```python
from build123d import *

# Parameters (mm, degrees)
F0_R     = 9
F0_R_2   = 1.45
F1_DEPTH = 2
F2_R     = 3
F2_R_2   = 1.5
F3_DEPTH = 15
F5_SIZE2 = 5
F5_SIZE  = 1
F6_DEPTH = 12


with BuildPart() as f1:
    # F0 (on Top) → F1 (new body)
    with BuildSketch(Plane.XY):
        with Locations((-40.0538817048, 19.144397229)):
            Circle(F0_R)
        with Locations((-40.0538817048, 19.144397229)):
            Circle(F0_R_2, mode=Mode.SUBTRACT)
    extrude(amount=F1_DEPTH)

    # F2 (on face) → F3 (join)
    with BuildSketch(Plane.XY.offset(2)):
        with Locations((-40.0538817048, 19.144397229)):
            Circle(F2_R)
        with Locations((-40.0538817048, 19.144397229)):
            Circle(F2_R_2, mode=Mode.SUBTRACT)
    extrude(amount=F3_DEPTH)

    # F5
    f5_edges = [f1.edges().sort_by_distance(p)[0] for p in [
        (-43.053882, 19.144397, 17),
    ]]
    f5_side = f1.faces().sort_by_distance((-42.969029, 19.144397, 17))[0]
    chamfer(f5_edges, length=F5_SIZE, length2=F5_SIZE2, reference=f5_side)

    # F4 (on face) → F6 (cut)
    with BuildSketch(Plane.XY.offset(17)):
        Polygon((-40.5538817048, 19.644397229), (-40.0538817048, 19.644397229), (-39.5538817048, 19.644397229), (-39.5538817048, 23.144397229), (-40.0538817048, 23.144397229), (-40.5538817048, 23.144397229), align=None)
        Polygon((-39.5538817048, 19.644397229), (-40.0538817048, 19.644397229), (-40.5538817048, 19.644397229), (-40.5538817048, 19.144397229), (-40.5538817048, 18.644397229), (-40.0538817048, 18.644397229), (-39.5538817048, 18.644397229), (-39.5538817048, 19.144397229), align=None)
        Polygon((-36.0538817048, 19.644397229), (-39.5538817048, 19.644397229), (-39.5538817048, 19.144397229), (-39.5538817048, 18.644397229), (-36.0538817048, 18.644397229), (-36.0538817048, 19.144397229), align=None)
        Polygon((-40.5538817048, 19.144397229), (-40.5538817048, 19.644397229), (-44.0538817048, 19.644397229), (-44.0538817048, 19.144397229), (-44.0538817048, 18.644397229), (-40.5538817048, 18.644397229), align=None)
        Polygon((-39.5538817048, 15.144397229), (-39.5538817048, 18.644397229), (-40.0538817048, 18.644397229), (-40.5538817048, 18.644397229), (-40.5538817048, 15.144397229), (-40.0538817048, 15.144397229), align=None)
    extrude(amount=-F6_DEPTH, mode=Mode.SUBTRACT)


solid = f1.part
```
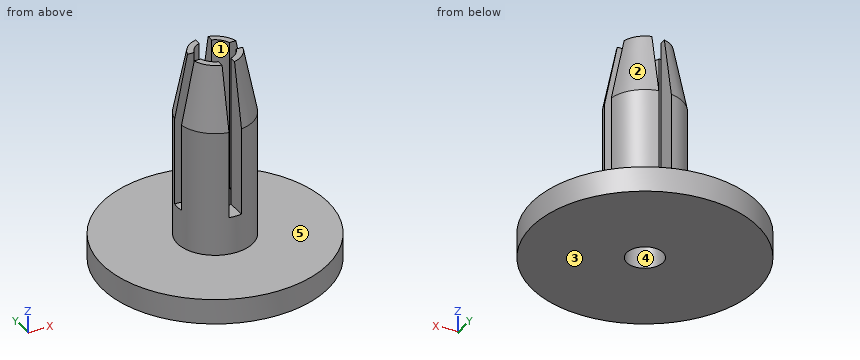
Model file for the job. Use its own axes, mm. Face numbers are marked on the shaded views. A direction names the side the tool comes from. Coordinates: 2 decimals unless noted, no trailing zeros. Loops run counter-clockwise (first coordinate to the right, second up) from the corner with the lowest first, then second, coordinate; pieces in that order, holes last. Notation, with made-up numbers: M 48,77.25 L 61,77.25 A29 cw 61,107.25 Z; hole C -12,88.5 d4. An arc over 180 degrees is marked long. Use CSV: the item, a comma, the result in double quotes. Start each with the question number.
1. Probe probe 1 along Z at (x, y) = (-38.75, 12); probe 2 along Y at (x, z) = (-41.25, 4.25); probe 3 along X at (y, z) = (17.75, 15.25). List the from-to ranges inside material, lowest first. Write a range as [from, to].
2. Band-saw the part on C-C, the plane y = 12.75. List the corners of the cut face in (x, z), then the cut area to 3 significant figures.
3. Tool access for the marked faces 4 and 5: list every direction of +Z, -Z, +X, -X, +Y, -Y with a clear straight run to the whole face (end or side of a thin tool).
4. Band-saw the part on A-A, the plane z = 10. List the corners of the cut face in (x, y), then the cut area to 3 significant figures.
5. Band-saw the part on D-D, the plane z = 14.25. List the corners of the cut face in (x, y), then the cut area to 3 significant figures.
6. Flat gauge pins, fed straight in: pin 1 (0.5 mm diameter, centred on x = -38, z = 8.5, fed in from -Y); pin 2 (8 mm diameter, centred on x = -45.5, z = 2.5, fed in from -Y); pin 3 (0.8 mm diameter, centred on x = -40, y = 17.5, fed in from +Z). Where does each tip first touch, or does it go through?
7. Band-saw the part on B-B, the plane x = -40.25. List the corners of the cut face in (y, z).
8. Two-plate mould, pull along Y, no slides. Class the marked faces 1, 2 and 3: pulls with the +Y half, pulls with the -Y half, needs draft (parallel to the pull), parting line crosses it, or undercut.
Entries:
1,probe 1,"z = [0, 2]"
1,probe 2,"y = [16.39, 18.24], [20.05, 21.9]"
1,probe 3,"x = [-41.95, -40.61], [-39.5, -38.16]"
2,outline,"M -46.39,0 L -33.72,0 L -33.72,2 L -46.39,2 Z"
2,area,"25.3 mm2"
3,face 4,"+Z, -Z"
3,face 5,"+Z"
4,outline,"M -43.01,18.64 A3 ccw -40.55,16.19 L -40.55,17.73 A1.5 cw -41.47,18.64 Z; M -43.01,19.64 L -41.47,19.64 A1.5 cw -40.55,20.56 L -40.55,22.1 A3 ccw Z; M -39.55,16.19 A3 ccw -37.1,18.64 L -38.64,18.64 A1.5 cw -39.55,17.73 Z; M -39.55,20.56 A1.5 cw -38.64,19.64 L -37.1,19.64 A3 ccw -39.55,22.1 Z"
4,area,"15.1 mm2"
5,outline,"M -42.55,18.64 A2.55 ccw -40.55,16.64 L -40.55,17.73 A1.5 cw -41.47,18.64 Z; M -42.55,19.64 L -41.47,19.64 A1.5 cw -40.55,20.56 L -40.55,21.64 A2.55 ccw Z; M -39.55,16.64 A2.55 ccw -37.55,18.64 L -38.64,18.64 A1.5 cw -39.55,17.73 Z; M -39.55,20.56 A1.5 cw -38.64,19.64 L -37.55,19.64 A2.55 ccw -39.55,21.64 Z"
5,area,"9.11 mm2"
6,pin 1,"stops at y = 16.75"
6,pin 2,"stops at y = 10.27"
6,pin 3,"stops at z = 5"
7,outline,"M 10.15,0 L 17.71,0 L 17.71,2 L 17.66,2 L 17.66,5 L 16.15,5 L 16.15,2 L 10.15,2 Z; M 20.58,0 L 28.14,0 L 28.14,2 L 22.14,2 L 22.14,5 L 20.63,5 L 20.63,2 L 20.58,2 Z"
8,face 1,"undercut"
8,face 2,"pulls with the +Y half"
8,face 3,"needs draft"
